Check sheet for the modelled part. Datum: model origin and axes. Units: mm. Face numbers are marked on the shaded views. A direction names the side the tool comes from. Coordinates: 2 decimals unless noted, no trailing zeros. Write each loop counter-clockwise with the first axis right and the second up, starting at its lowest first coordinate (ties: lowest second). Pieces come first, ordered by that corner, then holes. Notation, with made-up numbers: (77, 23) - (130, 23) arc R11 cw to (130, 44) - close; hole circle Ø8 at (9.25, 31). An arc over 180 degrees is marked (long way). Use one line per item in the form item = value. Start each with the question number.
1. Cross-section at B-B on y = 5.2. Record the boundary of the cut face in (x, z).
2. Cross-section at D-D on x = -7.5. Record the boundary of the cut face in (y, z).
3. Tool access check on the marked faces 1, 2, 3, 4 and 5. Record the directions out of +Z, -Z, +X, -X, +Y, -Y that give a thin tool (end or side, any length) a straight path to the whole face; none if there is none.
4. Scan lines: line 1 along Z through (x, y) = (-5.25, 3.75); line 2 along X through (y, z) = (1.3, -1); line 3 along Z through (x, y) = (1.75, 3.7). Record each from-to range of solid material in increasing order.
5. Go/stop test with flat-tipped pins: pin 1 Ø2 at (x, z) = (9.5, -6.5) entering from +Y; pin 2 Ø3 at (x, y) = (-2, 4) entering from -Z; pin 3 Ø8 at (x, z) = (6.5, -8.5) entering from +Y. Record where each tip stops, or that it passes through.
6. Cross-section at C-C on z = 1.5. Record the boundary of the cut face in (x, y), then the cut area to 3 significant figures.
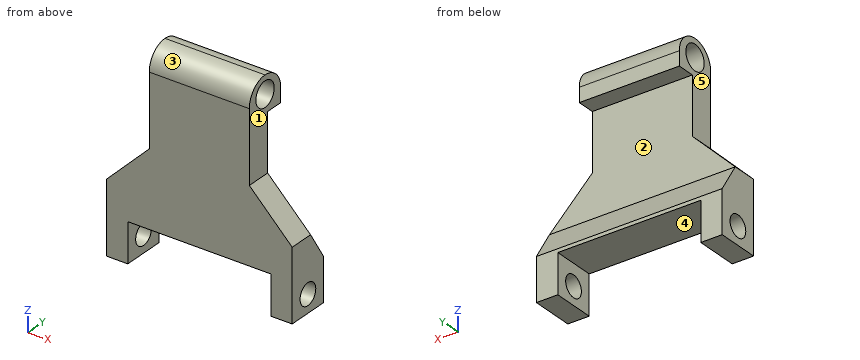
```python
from build123d import *

# Parameters (mm, degrees)
RESSALTO_EXTRUS_O1_DEPTH = 6
CORTE_EXTRUS_O1_DEPTH    = 33.58872513
ESBO_O5_R                = 1.75
CORTE_EXTRUS_O2_DEPTH    = 29.036137494
FILETE1_R                = 3
ESBO_O6_W                = 20
ESBO_O6_H                = 5.5
CORTE_EXTRUS_O3_DEPTH    = 24.558968686
ESBO_O7_R                = 1.5
CORTE_EXTRUS_O4_DEPTH    = 33.58872513


with BuildPart() as part:
    # Esboço1 → Ressalto-extrusão1 (new body)
    with BuildSketch(Plane(origin=(0, 0, 0), x_dir=(1, 0, 0), z_dir=(0, 1, 0))):
        Polygon((7, -10.291044776), (-7, -10.291044776), (-7, 2.708955224), (-13, 8.708955224), (-13, 18.708955224), (13, 18.708955224), (13, 8.708955224), (7, 2.708955224), align=None)
    extrude(amount=RESSALTO_EXTRUS_O1_DEPTH)

    # Esboço4 → Corte-extrusão1 (cut, through all)
    with BuildSketch(Plane.ZY.offset(13)):
        Polygon((-12.708955224, 6), (-8.708955224, 3.5), (5.291044776, 3.5), (5.291044776, 13.308893529), (-12.708955224, 13.308893529), align=None)
    extrude(amount=-CORTE_EXTRUS_O1_DEPTH, mode=Mode.SUBTRACT)

    # Esboço5 → Corte-extrusão2 (cut, through all)
    with BuildSketch(Plane.ZY.offset(7)):
        with Locations((7.791044776, 3)):
            Circle(ESBO_O5_R)
    extrude(amount=-CORTE_EXTRUS_O2_DEPTH, mode=Mode.SUBTRACT)

    # Filete1
    filete1_edges = [part.edges().sort_by_distance(p)[0] for p in [
        (0, 0, 10.291044776),
        (0, 6, 10.291044776),
    ]]
    fillet(filete1_edges, radius=FILETE1_R - 0.0001)  # a hair under: the kernel refuses the full size

    # Esboço6 → Corte-extrusão3 (cut, through all)
    with BuildSketch(Plane(origin=(0, 6, 0), x_dir=(1, 0, 0), z_dir=(0, 1, 0))):
        with Locations((0, 15.958955224)):
            Rectangle(ESBO_O6_W, ESBO_O6_H)
    extrude(amount=-CORTE_EXTRUS_O3_DEPTH, mode=Mode.SUBTRACT)

    # Esboço7 → Corte-extrusão4 (cut, through all)
    with BuildSketch(Plane.ZY.offset(13)):
        with Locations((-16.208955224, 3)):
            Circle(ESBO_O7_R)
    extrude(amount=-CORTE_EXTRUS_O4_DEPTH, mode=Mode.SUBTRACT)


solid = part.part
```
Final values:
q1.outline = (-13, -18.71) - (-10, -18.71) - (-10, -13.21) - (10, -13.21) - (10, -18.71) - (13, -18.71) - (13, -11.43) - (-13, -11.43) - close; (-7, 5.29) - (7, 5.29) - (7, 9.33) - (-7, 9.33) - close
q2.outline = (0, -13.21) - (6, -13.21) - (6, -12.71) - (3.5, -8.71) - (3.5, -3.21) - (0, -3.21) - close
q3.face_1 = +Z, +X, +Y, -Y
q3.face_2 = +X, -X, +Y
q3.face_3 = +Z, +X, -X, -Y
q3.face_4 = -Z, +Y, -Y
q3.face_5 = +Z, -X, +Y, -Y
q4.line_1 = -13.21 to -9.11, 5.29 to 6.21, 9.37 to 10.2
q4.line_2 = -7 to 7
q4.line_3 = -13.21 to -9.03, 5.29 to 6.19, 9.39 to 10.21
q5.pin_1 = 3.5
q5.pin_2 = -13.21
q5.pin_3 = 5.87
q6.outline = (-7, 0) - (7, 0) - (7, 3.5) - (-7, 3.5) - close
q6.area = 49.0 mm²
